from build123d import *

# Parameters (mm, degrees)
F1_DEPTH = 12.7
F2_R     = 25.4
F3_R     = 25.4


with BuildPart() as f1:
    # F0 (on Front) → F1 (new body)
    with BuildSketch(Plane.XZ):
        with BuildLine():
            ThreePointArc((-34.945074, 46.127506), (-51.027386, 53.720366), (-58.223099, 69.984252))
            ThreePointArc((-58.223099, 69.984252), (-62.31415, 31.507538), (-49.854971, -5.125275))
            Line((-49.854971, -5.125275), (11.182429, -5.125275))
            ThreePointArc((11.182429, -5.125275), (23.71529, 32.192738), (19.103313, 71.28796))
            ThreePointArc((19.103313, 71.28796), (13.57664, 58.599304), (0, 55.912126))
            ThreePointArc((0, 55.912126), (-14.268957, 71.506168), (-23.762649, 90.391271))
            ThreePointArc((-23.762649, 90.391271), (-32.331491, 69.011631), (-34.945074, 46.127506))
        make_face()
    extrude(amount=F1_DEPTH)

    # F2
    f2_edges = [f1.edges().sort_by_distance(p)[0] for p in [
        (-49.854971, -6.35, -5.125275),
    ]]
    fillet(f2_edges, radius=F2_R)

    # F3
    f3_edges = [f1.edges().sort_by_distance(p)[0] for p in [
        (11.182429, -6.35, -5.125275),
    ]]
    fillet(f3_edges, radius=F3_R)


solid = f1.part
Part model, mm, in its own coordinate system. A direction names the side the tool comes from. Give positions to 0.01 mm unless a question says otherwise; leave off trailing zeros. Order: outer loops, then holes, each group sorted by start corner. A loop starts at its lowest first (then second) coordinate and runs counter-clockwise, first axis right, second up. Notation, with made-up numbers: (79, 31.25) -> (114, 31.25) arc R16 ccw to (114, 36.25) -> close; hole circle Ø10 at (-34.75, -33.75). An arc over 180 degrees is marked (long way). Use one line per item in the form item = value.
(1) Saw through at A-A (y = -5.5). Write the cut outline in (x, z).
Solution:
outline = (-58.22, 69.98) arc R89.91 ccw to (-57.88, 11.93) arc R25.4 ccw to (-33.89, -5.13) -> (-4.78, -5.13) arc R25.4 ccw to (19.21, 11.93) arc R89.91 ccw to (19.1, 71.29) arc R14.92 cw to (0, 55.91) arc R77.04 cw to (-23.76, 90.39) arc R86.37 ccw to (-34.95, 46.13) arc R25.47 cw to start
(2) Drill centre lines: line 1 (X direction, y = -3, z = 56.5); line 2 (X direction, y = -3.5, z = 60.5); line 3 (X direction, y = -1.5, z = 54). Where is each one in solid material? Low to high. Write a range as from..to.
Solution:
line_1 = -61.6..-53.38, -34.53..-0.7, 10.08..22.93
line_2 = -60.83..-55.77, -34.03..-5.06, 15.54..22.16
line_3 = -61.99..-51.3, -34.74..23.32
(3) Flat gauge pins, fed straight in: P1, Ø12, axis at x = -51, z = 74, coming from the +Y side; P2, Ø2, axis at y = -4.5, z = 70, coming from the -X side; P3, Ø6, axis at x = -14.5, y = -1.5, coming from the +Z side; P4, Ø2, axis at x = -43, y = -4, coming from the -Z side. Where does each tip first touch, or does it go through?
Solution:
P1 = through
P2 = -58.55
P3 = 76.61
P4 = -3.8
(4) Tool access for faces 5 (the face through (-20, -12.7, 33)), 6 (the face through (-14.1, -6.26, 71.26)): list every direction of +Z, -Z, +X, -X, +Y, -Y with a clear straight run to the whole face (end or side of a thin tool).
Solution:
face_5 = +Z, -Z, +X, -X, -Y
face_6 = +Z, +Y, -Y
(5) Pull direction X, two halves, no side cores. Call faces 1 (the face through (-50.85, -6.26, 53.54)), 2 (the face through (-32.25, -6.26, 69.33)), 3 (the face through (9.754, -6.439, -0.553)), 4 (the face through (-62.867, -6.261, 41.343)): +X half, -X half, draft (parallel to the pull), parting line (faces both ways), or undercut.
Solution:
face_1 = undercut
face_2 = undercut
face_3 = +X half
face_4 = -X half
(6) Saw through at B-B (x = 5). Write the cut outline in (y, z).
Solution:
outline = (-12.7, -3.17) -> (0, -3.17) -> (0, 55.32) -> (-12.7, 55.32) -> close
(7) Saw through at C-C (z = 80). Write the cut outline in (x, y), then the cut area to 3 significant figures.
Solution:
outline = (-28.76, -12.7) -> (-19.35, -12.7) -> (-19.35, 0) -> (-28.76, 0) -> close
area = 119 mm²
